from build123d import *

# Parameters (mm, degrees)
F1_DEPTH = 6
F2_R     = 1
F3_R     = 1


with BuildPart() as f1:
    # F0 (on Top) → F1 (new body)
    with BuildSketch(Plane.XY):
        with BuildLine():
            ThreePointArc((-5.2915026221, -1.5), (0, -5.5), (5.2915026221, -1.5))
            Line((5.2915026221, -1.5), (2.5980762114, -1.5))
            ThreePointArc((2.5980762114, -1.5), (2.1861406616, -2.0544558909), (1.6583123952, -2.5))
            ThreePointArc((1.6583123952, -2.5), (0, -3), (-1.6583123952, -2.5))
            ThreePointArc((-1.6583123952, -2.5), (-2.1861406616, -2.0544558909), (-2.5980762114, -1.5))
            Line((-2.5980762114, -1.5), (-5.2915026221, -1.5))
        make_face()
        with BuildLine():
            ThreePointArc((-5.2915026221, -1.5), (-5.5, 0), (-5.2915026221, 1.5))
            Line((-5.2915026221, 1.5), (-15, 1.5))
            Line((-15, 1.5), (-15, -1.5))
            Line((-15, -1.5), (-5.2915026221, -1.5))
        make_face()
        with BuildLine():
            Line((-2.5980762114, 1.5), (-5.2915026221, 1.5))
            ThreePointArc((-5.2915026221, 1.5), (-5.5, 0), (-5.2915026221, -1.5))
            Line((-5.2915026221, -1.5), (-2.5980762114, -1.5))
            ThreePointArc((-2.5980762114, -1.5), (-3, 0), (-2.5980762114, 1.5))
        make_face()
        with BuildLine():
            ThreePointArc((5.2915026221, 1.5), (5.4476262914, 0.7572105316), (5.5, 0))
            ThreePointArc((5.5, 0), (5.4476262914, -0.7572105316), (5.2915026221, -1.5))
            Line((5.2915026221, -1.5), (15, -1.5))
            Line((15, -1.5), (15, 1.5))
            Line((15, 1.5), (5.2915026221, 1.5))
        make_face()
        with BuildLine():
            ThreePointArc((5.2915026221, -1.5), (5.4476262914, -0.7572105316), (5.5, 0))
            ThreePointArc((5.5, 0), (5.4476262914, 0.7572105316), (5.2915026221, 1.5))
            Line((5.2915026221, 1.5), (2.5980762114, 1.5))
            ThreePointArc((2.5980762114, 1.5), (2.8977774789, 0.7764571353), (3, 0))
            ThreePointArc((3, 0), (2.8977774789, -0.7764571353), (2.5980762114, -1.5))
            Line((2.5980762114, -1.5), (5.2915026221, -1.5))
        make_face()
        with BuildLine():
            Line((2.5980762114, 1.5), (5.2915026221, 1.5))
            ThreePointArc((5.2915026221, 1.5), (0, 5.5), (-5.2915026221, 1.5))
            Line((-5.2915026221, 1.5), (-2.5980762114, 1.5))
            ThreePointArc((-2.5980762114, 1.5), (-2.1861406616, 2.0544558909), (-1.6583123952, 2.5))
            ThreePointArc((-1.6583123952, 2.5), (0, 3), (1.6583123952, 2.5))
            ThreePointArc((1.6583123952, 2.5), (2.1861406616, 2.0544558909), (2.5980762114, 1.5))
        make_face()
        with BuildLine():
            Line((-1.6583123952, 2.5), (1.6583123952, 2.5))
            ThreePointArc((1.6583123952, 2.5), (0, 3), (-1.6583123952, 2.5))
        make_face()
        with BuildLine():
            ThreePointArc((-1.6583123952, -2.5), (0, -3), (1.6583123952, -2.5))
            Line((1.6583123952, -2.5), (-1.6583123952, -2.5))
        make_face()
    extrude(amount=F1_DEPTH)

    # F2
    f2_edges = [f1.edges().sort_by_distance(p)[0] for p in [
        (15, -1.5, 3),
        (-15, -1.5, 3),
        (15, 1.5, 3),
        (-15, 1.5, 3),
    ]]
    fillet(f2_edges, radius=F2_R)

    # F3
    f3_edges = [f1.edges().sort_by_distance(p)[0] for p in [
        (5.291503, -1.5, 3),
        (-5.291503, -1.5, 3),
        (-5.291503, 1.5, 3),
        (5.291503, 1.5, 3),
        (-1.658312, 2.5, 3),
        (1.658312, -2.5, 3),
        (1.658312, 2.5, 3),
        (-1.658312, -2.5, 3),
    ]]
    fillet(f3_edges, radius=F3_R)


solid = f1.part
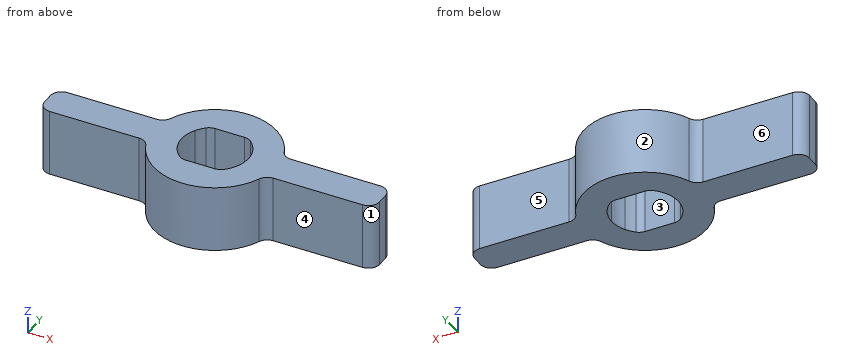
CAD build for the part. Positions are in the model's coordinates, mm. Face numbers are marked on the shaded views. A direction names the side the tool comes from. Coordinates: 2 decimals unless noted, no trailing zeros. Write each loop counter-clockwise with the first axis right and the second up, starting at its lowest first coordinate (ties: lowest second). Pieces come first, ordered by that corner, then holes. Notation, with made-up numbers: M -1,62.25 L 39,62.25 A10 ccw 39,66.25 Z; hole C -23.5,20 d1. An arc over 180 degrees is marked long. Answer as a JSON object with one key per item and string values. Group by question number.
1) Saw through at A-A (z = 3.2). Write the cut outline in (x, y), plus the area to 3 significant figures.
2) Tool access for the marked faces 4, 5 and 6: list every direction of +Z, -Z, +X, -X, +Y, -Y with a clear straight run to the whole face (end or side of a thin tool).
3) Saw through at B-B (x = -10.5). Write the cut outline in (y, z), plus the area to 3 significant figures.
4) Mould opens along Y. For the marked faces 1, 2 and 3 say: +Y half, -Y half, draft (parallel to the pull), parting line (faces both ways), or undercut.
5) Pin check, flat tips, straight feed: pin 1 Ø1.8 at (x, z) = (-11.5, 1.5) entering from +Y; pin 2 Ø2 at (x, z) = (7.5, 1.5) entering from -Y; pin 3 Ø1.5 at (y, z) = (-3, 3) entering from +X. Stop position of each tip, or through.
6) Saw through at C-C (y = -3.75). Write the cut outline in (x, z).
7) Wall check: line 1 (X direction, y = 0, z = 0.4); line 2 (Y direction, x = -9.75, z = 4.2); line 3 (X direction, y = 2, z = 5.15). Give the ranges that are in metal, low to high. Write a range as from..to.
Values follow:
{
 "1": {"outline": "M -15,-0.5 A1 ccw -14,-1.5 L -6,-1.5 A1 cw -5.08,-2.12 A5.5 ccw 5.08,-2.12 A1 cw 6,-1.5 L 14,-1.5 A1 ccw 15,-0.5 L 15,0.5 A1 ccw 14,1.5 L 6,1.5 A1 cw 5.08,2.12 A5.5 ccw -5.08,2.12 A1 cw -6,1.5 L -14,1.5 A1 ccw -15,0.5 Z; hole M -1.98,-2.25 A1 ccw -1.32,-2.5 L 1.32,-2.5 A1 ccw 1.98,-2.25 A3 ccw 1.98,2.25 A1 ccw 1.32,2.5 L -1.32,2.5 A1 ccw -1.98,2.25 A3 ccw Z", "area": "126 mm2"},
 "2": {"face 4": "+Z, -Z, +X, -Y", "face 5": "+Z, -Z, +X, +Y", "face 6": "+Z, -Z, -X, +Y"},
 "3": {"outline": "M -1.5,0 L 1.5,0 L 1.5,6 L -1.5,6 Z", "area": "18.0 mm2"},
 "4": {"face 1": "-Y half", "face 2": "+Y half", "face 3": "undercut"},
 "5": {"pin 1": "stops at y = 1.5", "pin 2": "stops at y = -1.5", "pin 3": "stops at x = 5.02"},
 "6": {"outline": "M -4.02,0 L 4.02,0 L 4.02,6 L -4.02,6 Z"},
 "7": {"line 1": "x = -15..-3, 3..15", "line 2": "y = -1.5..1.5", "line 3": "x = -5.13..-2.24, 2.24..5.13"}
}
